Part model, mm, in its own coordinate system. Face numbers are marked on the shaded views. A direction names the side the tool comes from. Coordinates: 2 decimals unless noted, no trailing zeros. Loops run counter-clockwise (first coordinate to the right, second up) from the corner with the lowest first, then second, coordinate; pieces in that order, holes last. Notation, with made-up numbers: (1, -30) -> (34, -30) arc R31 cw to (34, -1) -> close; hole circle Ø7 at (-33, -33.5). An arc over 180 degrees is marked (long way). One line per item, written item: value. Start each with the question number.
from build123d import *

# Parameters (mm, degrees)
F3_DEPTH = 10
F4_R     = 1.5
F5_DEPTH = 25
F6_R     = 1.5
F7_DEPTH = 25
F8_F1_R  = 0.4
F8_F2_R  = 0.4
F8_F3_R  = 0.4
F8_F4_R  = 0.4


# Not quite as in the source:
# - a feature names something its author has since deleted; it is built from what else it names


with BuildPart() as f1:
    # F0 (on Top) → F1 (revolve)
    with BuildSketch(Plane.XY):
        Polygon((22.5, 0.8), (22.5, 0), (37.5, 0), (7.5, 16.6666666667), (1.5, 16.6666666667), (1.5, 14.6888888889), (7.5, 14.6888888889), (32.5, 0.8), align=None)
    revolve(axis=Axis((0, 10, 0), (0, 1, 0)))

    # F2 (on face) → F3 (join)
    with BuildSketch(Plane.XZ):
        with BuildLine():
            Line((-31.9726445575, -10), (-31.9726445575, 10))
            ThreePointArc((-31.9726445575, 10), (-33.5, 0), (-31.9726445575, -10))
        make_face()
        with BuildLine():
            ThreePointArc((31.9726445575, -10), (33.5, 0), (31.9726445575, 10))
            Line((31.9726445575, 10), (31.9726445575, -10))
        make_face()
    extrude(amount=F3_DEPTH)

    # F4 (on face) → F5 (cut)
    with BuildSketch(Plane.YZ.offset(-31.9726445575)):
        with Locations((-5, 0)):
            Circle(F4_R)
    extrude(amount=-F5_DEPTH, mode=Mode.SUBTRACT)

    # F6 (on face) → F7 (cut)
    with BuildSketch(Plane(origin=(31.9726445575, 0, 0), x_dir=(0, -1, 0), z_dir=(-1, 0, 0))):
        with Locations((5, 0)):
            Circle(F6_R)
    extrude(amount=-F7_DEPTH, mode=Mode.SUBTRACT)

    # F8: fillet of radius 0.4 on 4 edges, made by hand

    # F8_f1
    f8_f1_edges = [f1.edges().sort_by_distance(p)[0] for p in [
        (31.9726445575, -5, 10),
    ]]
    fillet(f8_f1_edges, radius=F8_F1_R)

    # F8_f2
    f8_f2_edges = [f1.edges().sort_by_distance(p)[0] for p in [
        (31.9726445575, -5, -10),
    ]]
    fillet(f8_f2_edges, radius=F8_F2_R)

    # F8_f3
    f8_f3_edges = [f1.edges().sort_by_distance(p)[0] for p in [
        (-31.9726445575, -5, -10),
    ]]
    fillet(f8_f3_edges, radius=F8_F3_R)

    # F8_f4
    f8_f4_edges = [f1.edges().sort_by_distance(p)[0] for p in [
        (-31.9726445575, -5, 10),
    ]]
    fillet(f8_f4_edges, radius=F8_F4_R)


solid = f1.part
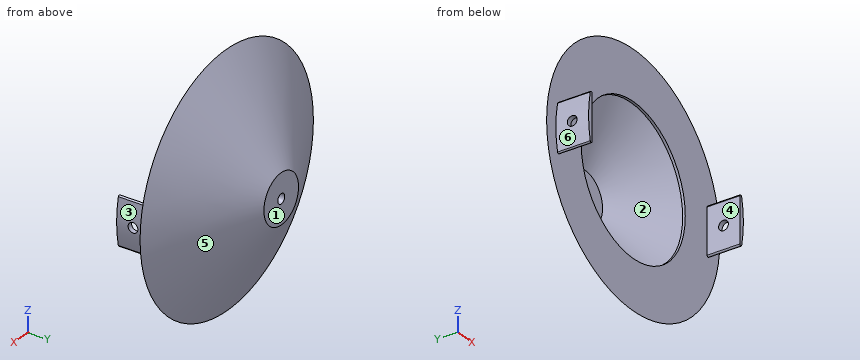
1) Slice it at B-B (x = 0). Give the cut face in (y, z).
2) Tool access for the marked faces 4, 5 and 6: list every direction of +Z, -Z, +X, -X, +Y, -Y with a clear straight run to the whole face (end or side of a thin tool).
3) Probe line 1 (X direction, y = -7, z = 4); line 2 (X direction, y = -3.5, z = 5); line 3 (Y direction, x = 8.5, z = 27). List the from-to ranges inside material, lowest first. Write a range as from..to.
4) Slice it at C-C (y = -5). Give the cut face in (x, z).
5) Slice it at A-A (z = 0). State how many separate pieces and enclosed holes the cut face has, then the cut area to 3 significant figures.
6) Pin check, flat tips, straight feed: pin 1 Ø5 at (x, z) = (7, -13.5) entering from -Y; pin 2 Ø8 at (x, z) = (-13, -13.5) entering from +Y; pin 3 Ø4 at (x, z) = (1.5, 27.5) entering from -Y. Stop position of each tip, or through.
7) Pull direction X, two halves, no side cores. Call the marked faces 1, 2 and 3: +X half, -X half, draft (parallel to the pull), parting line (faces both ways), or undercut.
8) Slice it at D-D (y = 2.75). Give the cut face in (x, z).
Check sheet entries:
1. outline: (0, -37.5) -> (16.67, -7.5) -> (16.67, -1.5) -> (14.69, -1.5) -> (14.69, -7.5) -> (0.8, -32.5) -> (0.8, -22.5) -> (0, -22.5) -> close; (0, 22.5) -> (0.8, 22.5) -> (0.8, 32.5) -> (14.69, 7.5) -> (14.69, 1.5) -> (16.67, 1.5) -> (16.67, 7.5) -> (0, 37.5) -> close
2. face 4: +Z, -Z, -Y
2. face 5: +Y
2. face 6: -X, -Y
3. line 1: x = -33.26..-31.97, 31.97..33.26
3. line 2: x = -33.12..-31.97, 31.97..33.12
3. line 3: y = 0..0.8, 3.13..5.11
4. outline: (-33.47, -1.5) arc R33.5 ccw to (-32.76, -6.98) arc R0.4 ccw to (-31.97, -6.9) -> (-31.97, -1.5) -> close; (-33.47, 1.5) -> (-31.97, 1.5) -> (-31.97, 6.9) arc R0.4 ccw to (-32.76, 6.98) arc R33.5 ccw to start; (31.97, -6.9) arc R0.4 ccw to (32.76, -6.98) arc R33.5 ccw to (33.47, -1.5) -> (31.97, -1.5) -> close; (31.97, 1.5) -> (33.47, 1.5) arc R33.5 ccw to (32.76, 6.98) arc R0.4 ccw to (31.97, 6.9) -> close
5. separate pieces: 4
5. enclosed holes: 0
5. area: 174 mm^2
6. pin 1: stops at y = 9.02
6. pin 2: stops at y = 12.64
6. pin 3: stops at y = 0
7. face 1: draft
7. face 2: undercut
7. face 3: +X half
8. outline: circle Ø65.1 at (0, 0); hole circle Ø57.98 at (0, 0)
